```python
from build123d import *

# Parameters (mm, degrees)
F0_R     = 1.5
F0_R_2   = 1.375
F0_R_3   = 1
F1_DEPTH = 3.5
F2_R     = 8


# Not quite as in the source:
# - a feature names something its author has since deleted; it is built from what else it names


with BuildPart() as f1:
    # F0 (on Top) → F1 (new body)
    with BuildSketch(Plane.XY):
        Polygon((-37, 91), (-37, 81), (-14, 59), (-14, 39), (-30, 27), (-30, -23), (-14, -35), (-14, -45), (-25, -55.1980390272), (-25, -93), (25, -93), (25, -55.1980390272), (14, -45), (14, -35), (30, -23), (30, 27), (14, 39), (14, 59), (37, 81), (37, 91), (25, 100), (-25, 100), align=None)
        with Locations((-20, -88)):
            Circle(F0_R, mode=Mode.SUBTRACT)
        with Locations((-19.5, -68.25)):
            Circle(F0_R, mode=Mode.SUBTRACT)
        with Locations((-25, -18)):
            Circle(F0_R_2, mode=Mode.SUBTRACT)
        with Locations((-25, 2)):
            Circle(F0_R_2, mode=Mode.SUBTRACT)
        with Locations((0, -88)):
            Circle(F0_R, mode=Mode.SUBTRACT)
        with Locations((20, -88)):
            Circle(F0_R, mode=Mode.SUBTRACT)
        with Locations((20.5, -68.25)):
            Circle(F0_R, mode=Mode.SUBTRACT)
        with Locations((25, -18)):
            Circle(F0_R_2, mode=Mode.SUBTRACT)
        with Locations((25, 2)):
            Circle(F0_R_2, mode=Mode.SUBTRACT)
        with Locations((-25, 22)):
            Circle(F0_R_2, mode=Mode.SUBTRACT)
        with Locations((-32, 86)):
            Circle(F0_R_2, mode=Mode.SUBTRACT)
        with Locations((-20, 95)):
            Circle(F0_R, mode=Mode.SUBTRACT)
        Polygon((27, 86), (27, 85.2728960546), (4, 63.2728960546), (4, 34), (20, 22), (20, -18), (4, -30), (4, -49.3654190662), (15, -59.5634580934), (15, -83), (-15, -83), (-15, -59.5634580934), (-4, -49.3654190662), (-4, -30), (-20, -18), (-20, 22), (-4, 34), (-4, 63.2728960546), (-27, 85.2728960546), (-27, 86), (-21.6666666667, 90), (21.6666666667, 90), align=None, mode=Mode.SUBTRACT)
        with Locations((25, 22)):
            Circle(F0_R_2, mode=Mode.SUBTRACT)
        with Locations((0, 95)):
            Circle(F0_R, mode=Mode.SUBTRACT)
        with Locations((20, 95)):
            Circle(F0_R, mode=Mode.SUBTRACT)
        with Locations((32, 86)):
            Circle(F0_R_2, mode=Mode.SUBTRACT)
        Polygon((4, 63.2728960546), (27, 85.2728960546), (27, 86), (21.6666666667, 90), (-21.6666666667, 90), (-27, 86), (-27, 85.2728960546), (-4, 63.2728960546), (-4, 34), (4, 34), align=None)
        Polygon((4, -49.3654190662), (4, -30), (-4, -30), (-4, -49.3654190662), (-15, -59.5634580934), (-15, -83), (15, -83), (15, -59.5634580934), align=None)
        with Locations((0, -39.6827095331)):
            Circle(F0_R_3, mode=Mode.SUBTRACT)
    extrude(amount=F1_DEPTH)

    # F2
    f2_edges = [f1.edges().sort_by_distance(p)[0] for p in [
        (4, -30, 1.75),
        (-4, -30, 1.75),
        (20, -18, 1.75),
        (-25, -93, 1.75),
        (25, -93, 1.75),
        (25, -55.198039, 1.75),
        (14, -45, 1.75),
        (-25, -55.198039, 1.75),
        (-14, -45, 1.75),
        (-14, -35, 1.75),
        (14, -35, 1.75),
        (30, -23, 1.75),
        (-30, -23, 1.75),
        (-20, -18, 1.75),
        (-20, 22, 1.75),
        (20, 22, 1.75),
        (4, 34, 1.75),
        (-4, 34, 1.75),
        (-30, 27, 1.75),
        (-14, 39, 1.75),
        (30, 27, 1.75),
        (14, 39, 1.75),
        (-14, 59, 1.75),
        (14, 59, 1.75),
        (37, 81, 1.75),
        (37, 91, 1.75),
        (25, 100, 1.75),
        (-25, 100, 1.75),
        (-37, 81, 1.75),
        (-37, 91, 1.75),
    ]]
    fillet(f2_edges, radius=F2_R)


solid = f1.part
```
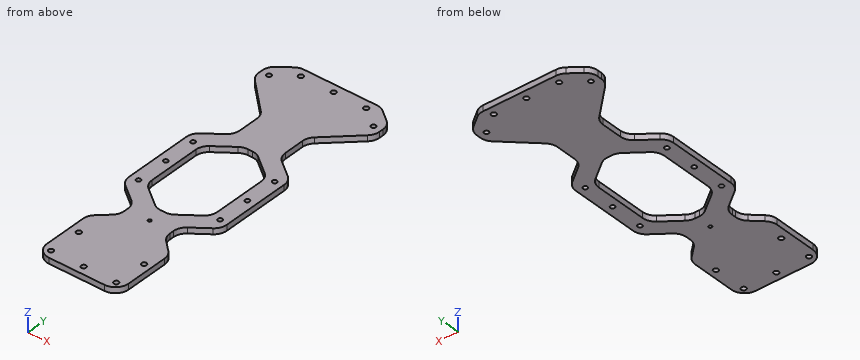
Design review of the part built by this model. Coordinates are the model's own, in mm. Give positions to 0.01 mm unless a question says otherwise; leave off trailing zeros. Order: outer loops, then holes, each group sorted by start corner. A loop starts at its lowest first (then second) coordinate and runs counter-clockwise, first axis right, second up. Notation, with made-up numbers: (70.25, 68) - (109.25, 68) arc R8 cw to (109.25, 75) - close; hole circle Ø7 at (20.5, -12). An arc over 180 degrees is marked (long way). Use a Markdown table: item, result. Add a question column.
(1) Add section A-A on x = 10.5. Give the boundary of the cut face in (y, z) (3 decimals), then the cut area to 3 significant figures.
(2) Add section B-B on y = 51.5. Give the boundary of the cut face in (x, z), then the cut area to 3 significant figures.
(3) Wall thickness on probe 1 along X at (y, z) = (-68.25, 2.05); probe 2 along Y at (x, z) = (0, 2.45); probe 3 along X at (y, z) = (86, 1.5) (3 decimals): over which ranges is each line inside the solid? List them lowest first. Write a range as [from, to].
(4) Add section C-C on z = 1.2. Give the number of separate pieces and of enclosed holes in the cut face, then the cut area to 3 significant figures.
(5) Clearance check with flat-ended pins moving along their axes: P1, Ø1.6, axis at x = -25, y = -18, coming from the +Z side; P2, Ø2, axis at y = 66, z = 1.5, coming from the -X side; P3, Ø1, axis at y = -76.5, z = 1, coming from the -X side; P4, Ø0.8, axis at y = -40.5, z = 1.5, coming from the -X side. State where each tip first meets the part, or that it passes through.
Report:
| question | item | result |
|---|---|---|
| 1 | outline | (-93, 0) - (-25.125, 0) - (-25.125, 3.5) - (-93, 3.5) - close; (29.125, 0) - (100, 0) - (100, 3.5) - (29.125, 3.5) - close |
| 1 | area | 486 mm² |
| 2 | outline | (-14, 0) - (14, 0) - (14, 3.5) - (-14, 3.5) - close |
| 2 | area | 98.0 mm² |
| 3 | probe 1 | x = [-25, -21], [-18, 19], [22, 25] |
| 3 | probe 2 | y = [-93, -89.5], [-86.5, -40.68], [-38.68, -30], [34, 93.5], [96.5, 100] |
| 3 | probe 3 | x = [-37, -33.375], [-30.625, 30.625], [33.375, 37] |
| 4 | separate pieces | 1 |
| 4 | enclosed holes | 18 |
| 4 | area | 7,300 mm² |
| 5 | P1 | passes through |
| 5 | P2 | stops at x = -22.36 |
| 5 | P3 | stops at x = -25 |
| 5 | P4 | stops at x = -14 |
